Verification items for the finished model (mm, model axes). A direction names the side the tool comes from. Round coordinates to 2 decimals unless told otherwise and drop trailing zeros. Loops run counter-clockwise (first coordinate to the right, second up) from the corner with the lowest first, then second, coordinate; pieces in that order, holes last. Notation, with made-up numbers: (-27, -25.5) - (9, -25.5) arc R16 cw to (9, -17.5) - close; hole circle Ø1 at (19.25, 13.5). An arc over 180 degrees is marked (long way). Use CSV: the item, a comma, the result in double quotes.
```python
from build123d import *

# Parameters (mm, degrees)
F0_W     = 110
F0_H     = 15
F1_DEPTH = 5
F2_R     = 4
F3_DEPTH = 33.5


with BuildPart() as f1:
    # F0 (on Front) → F1 (new body)
    with BuildSketch(Plane.XZ):
        with Locations((1.137998, 4.555882)):
            Rectangle(F0_W, F0_H)
    extrude(amount=F1_DEPTH)

    # F2 (on face) → F3 (join)
    with BuildSketch(Plane.XZ.offset(5)):
        with Locations((0, 2.855882)):
            Circle(F2_R)
        with BuildLine():
            Line((-48.680253, -2.944118), (-46.780253, -2.944118))
            ThreePointArc((-46.780253, -2.944118), (-48.680253, -1.044118), (-50.580253, -2.944118))
            Line((-50.580253, -2.944118), (-48.680253, -2.944118))
        make_face()
        with Locations((-45.862002, 4.686209)):
            Circle(F2_R)
        with Locations((45.862002, 4.686209)):
            Circle(F2_R)
        with BuildLine():
            ThreePointArc((50.580253, -2.944118), (48.680253, -1.044118), (46.780253, -2.944118))
            Line((46.780253, -2.944118), (50.580253, -2.944118))
        make_face()
    extrude(amount=F3_DEPTH)

    # F4: F1 across face


with BuildPart() as f1_1:
    add(f1.part)
    add(f1.part.mirror(Plane(origin=(-45.862002, -38.5, 4.686209), x_dir=(1, 0, 0), z_dir=(0, -1, 0))))


solid = f1_1.part
```
1) Gauge pin test, flat ends, axial feed: pin 1 Ø12 at (x, y) = (-34.5, -20.5) entering from +Z; pin 2 Ø7.5 at (x, z) = (-1.5, 7) entering from +Y. Record the tip position at first contact, or that the pin passes through.
Returned:
pin 1,"passes through"
pin 2,"stops at y = 0"
2) Access from +Z, -Z, +X, -X, +Y, -Y to the whole of each face (thin tool, end or side, straight path). Record for faces 1 (the face through (0, -73, -2.944)), 2 (the face through (48.722, -38.969, -1.045)).
Returned:
face 1,"-Z, +X, -X, +Y, -Y"
face 2,"none"
3) Cross-section at A-A, the plane x = -28.5. Record the cut outline in (y, z), then the cut area to 3 significant figures.
Returned:
outline,"(-77, -2.94) - (-72, -2.94) - (-72, 12.06) - (-77, 12.06) - close; (-5, -2.94) - (0, -2.94) - (0, 12.06) - (-5, 12.06) - close"
area,"150 mm²"
4) Thickness scan on probe 1 along Y at (x, z) = (46, -0.5); probe 2 along X at (y, z) = (-18.5, 6); probe 3 along X at (y, z) = (-33, 3.5). Record the ranges inside material, lowest first. Write a range as [from, to].
Returned:
probe 1,"y = [-77, -72], [-5, 0]"
probe 2,"x = [-49.64, -42.08], [-2.47, 2.47], [42.08, 49.64]"
probe 3,"x = [-49.68, -42.04], [-3.95, 3.95], [42.04, 49.68]"
5) Cross-section at D-D, the plane x = 0. Record the cut outline in (y, z).
Returned:
outline,"(-77, -2.94) - (-72, -2.94) - (-72, -1.14) - (-5, -1.14) - (-5, -2.94) - (0, -2.94) - (0, 12.06) - (-5, 12.06) - (-5, 6.86) - (-72, 6.86) - (-72, 12.06) - (-77, 12.06) - close"
6) Cross-section at B-B, the plane z = 10.5. Record the cut outline in (x, y).
Returned:
outline,"(-53.86, -77) - (56.14, -77) - (56.14, -72) - (-53.86, -72) - close; (-53.86, -5) - (56.14, -5) - (56.14, 0) - (-53.86, 0) - close"
7) Mould release check, pull along X, two halves, no side actions. Record for faces 3 (the face through (0, -2, 12.056)), 4 (the face through (-53.862, -2, 4)), 5 (the face through (0, -72, 8)), 6 (the face through (-48.638, -38.969, -1.045)): +X half, -X half, draft (parallel to the pull), parting line (faces both ways), or undercut.
Returned:
face 3,"draft"
face 4,"-X half"
face 5,"undercut"
face 6,"undercut"
8) Cross-section at C-C, the plane y = -62. Record the cut outline in (x, z), then the cut area to 3 significant figures.
Returned:
outline,"(-50.58, -2.94) - (-46.78, -2.94) arc R1.9 ccw to start; circle Ø8 at (-45.86, 4.69); circle Ø8 at (0, 2.86); circle Ø8 at (45.86, 4.69); (46.78, -2.94) - (50.58, -2.94) arc R1.9 ccw to start"
area,"162 mm²"
